Model file for the job. Use its own axes, mm. Face numbers are marked on the shaded views. A direction names the side the tool comes from. Give positions to 0.01 mm unless a question says otherwise; leave off trailing zeros. Loops run counter-clockwise (first coordinate to the right, second up) from the corner with the lowest first, then second, coordinate; pieces in that order, holes last. Notation, with made-up numbers: M 52,83 L 106,83 A20 ccw 106,118 Z; hole C 35.25,-32 d6. An arc over 180 degrees is marked long. Answer in a Markdown table with one row per item.
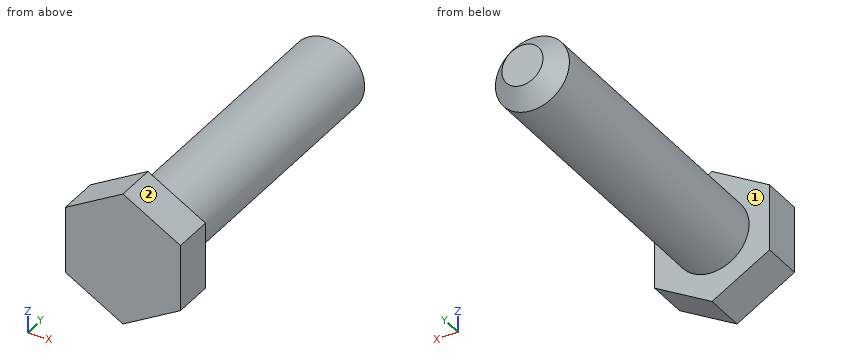
Autodesk Inventor part; units mm, degrees
ref_plane "YZ Plane" through (0, 0, 0) normal (1, 0, 0) x (0, 1, 0)
ref_plane "XZ Plane" through (0, 0, 0) normal (0, 1, 0) x (-1, 0, 0)
ref_plane "XY Plane" through (0, 0, 0) normal (0, 0, 1) x (1, 0, 0)
sketch "Sketch1" plane through (0, 0, 0) normal (0, 1, 0) x (-1, 0, 0)
  line L0 (7.5201, 21.3562) -> (14.5201, 17.3147)
  line L1 (14.5201, 17.3147) -> (14.5201, 9.2318)
  line L2 (14.5201, 9.2318) -> (7.5201, 5.1904)
  line L3 (7.5201, 5.1904) -> (0.5201, 9.2318)
  line L4 (0.5201, 9.2318) -> (0.5201, 17.3147)
  line L5 (0.5201, 17.3147) -> (7.5201, 21.3562)
  point P0 (7.5201, 13.2733)
  dimension "d0" = 14
extrude "Extrusion1" add sketch "Sketch1" along normal blind 5
sketch "Sketch2" plane through (0, 5, 0) normal (0, 1, 0) x (1, 0, 0)
  line L0 (-14.5201, -17.3147) -> (-7.5201, -21.3562)
  line L1 (-7.5201, -21.3562) -> (-0.5201, -17.3147)
  line L2 (-0.5201, -17.3147) -> (-0.5201, -9.2318)
  line L3 (-0.5201, -9.2318) -> (-7.5201, -5.1904)
  line L4 (-7.5201, -5.1904) -> (-14.5201, -9.2318)
  line L5 (-14.5201, -9.2318) -> (-14.5201, -17.3147)
  line L6 (-14.5201, -13.2733) -> (-0.5201, -13.2733) construction
  circle A0 centre (-7.5201, -13.2733) radius 4.5
  dimension "d3" = 9
extrude "Extrusion2" add sketch "Sketch2" along normal blind 38 contours A0
chamfer "Chamfer1" distance 2 angle 45 1 edges at (-12.0201, 43, 13.2733)
properties part number "perno_38"
Q1. Probe probe 1 along Y at (x, z) = (-1, 17); probe 2 along Z at (x, y) = (-3.5, 15); probe 3 along X at (y, z) = (31, 16). List the from-to ranges inside material, lowest first.
Reported:
| item | result |
|---|---|
| probe 1 | 0 to 5 |
| probe 2 | 11.25 to 15.3 |
| probe 3 | -11.1 to -3.94 |
Q2. Saw through at A-A (y = 35.5). Give the cut face in (x, z).
Reported:
| item | result |
|---|---|
| outline | C -7.52,13.27 d9 |
Q3. Saw through at B-B (x = -1.5). Give the cut face in (y, z), and give its area (3 significant figures).
Reported:
| item | result |
|---|---|
| outline | M 0,8.67 L 5,8.67 L 5,17.88 L 0,17.88 Z |
| area | 46.1 mm² |
Q4. Drop flat-ended pins along their axis: pin 1 (5 mm diameter, centred on x = -13, y = 4.5, fed in from +Z); pin 2 (4 mm diameter, centred on x = -4.5, z = 19.5, fed in from +Y); pin 3 (4 mm diameter, centred on x = -12.5, y = 14, fed in from +Z); pin 4 (4 mm diameter, centred on x = -7, z = 10, fed in from +Y). Give the stop position or say it passes through.
Reported:
| item | result |
|---|---|
| pin 1 | z = 19.64 |
| pin 2 | y = 5 |
| pin 3 | z = 16.65 |
| pin 4 | y = 43 |
Q5. Saw through at C-C (z = 8). Give the cut face in (x, y).
Reported:
| item | result |
|---|---|
| outline | M -12.39,0 L -2.65,0 L -2.65,5 L -12.39,5 Z |
Q6. 3-axis set-ups, long thin cutter, end or side, ignore diameter. For the marked faces 1 and 2: which of +Z, -Z, +X, -X, +Y, -Y reach the whole face in a straight line?
Reported:
| item | result |
|---|---|
| face 1 | +Y |
| face 2 | +Z, +X, +Y, -Y |
